```python
from build123d import *

# Parameters (mm, degrees)
SKETCH_1_W      = 60
SKETCH_1_H      = 60
EXTRUDE_1_DEPTH = 3
HOLE_WIZARD_1_D = 3
SKETCH_5_W      = 2
SKETCH_5_H      = 60
EXTRUDE_2_DEPTH = 23
SKETCH_6_W      = 60
SKETCH_6_H      = 3
EXTRUDE_3_DEPTH = 7
HOLE_WIZARD_2_D = 3.5
EXTRUDE_4_DEPTH = 3
EXTRUDE_5_DEPTH = 3


with BuildPart() as part:
    # 草图1 → 凸台-拉伸1 (new body)
    with BuildSketch(Plane(origin=(0, 0, 0), x_dir=(1, 0, 0), z_dir=(0, 1, 0))):
        Rectangle(SKETCH_1_W, SKETCH_1_H)
    extrude(amount=EXTRUDE_1_DEPTH)

    # 孔1 (through all)
    with Locations(Plane(origin=(0, 3, 0), x_dir=(1, 0, 0), z_dir=(0, 1, 0))):
        with Locations((-21.5, 21.5), (21.5, 21.5), (-21.5, -21.5), (21.5, -21.5)):
            Hole(HOLE_WIZARD_1_D / 2)

    # 草图5 → 凸台-拉伸2 (add)
    with BuildSketch(Plane(origin=(0, 3, 0), x_dir=(1, 0, 0), z_dir=(0, 1, 0))):
        with Locations((29, 0)):
            Rectangle(SKETCH_5_W, SKETCH_5_H)
        with Locations((-29, 0)):
            Rectangle(SKETCH_5_W, SKETCH_5_H)
    extrude(amount=EXTRUDE_2_DEPTH)

    # 草图6 → 凸台-拉伸3 (add)
    with BuildSketch(Plane(origin=(30, 0, 0), x_dir=(0, 0, -1), z_dir=(1, 0, 0))):
        with Locations((0, 24.5)):
            Rectangle(SKETCH_6_W, SKETCH_6_H)
    extrude_3 = extrude(amount=EXTRUDE_3_DEPTH)

    # 孔2 (through all)
    with Locations(Plane(origin=(0, 26, 0), x_dir=(1, 0, 0), z_dir=(0, 1, 0))):
        with Locations((33.5, 25), (33.5, -25)):
            hole_wizard_2 = Hole(HOLE_WIZARD_2_D / 2)

    # 镜向1: 凸台-拉伸3, 孔2 across plane
    add(extrude_3.mirror(Plane.ZY))
    add(hole_wizard_2.mirror(Plane.ZY), mode=Mode.SUBTRACT)

    # 草图11 → 凸台-拉伸4 (add)
    with BuildSketch(Plane(origin=(0, 0, -30), x_dir=(-1, 0, 0), z_dir=(0, 0, -1))):
        Polygon((-37, 26), (-28, 26), (-28, 3), (28, 3), (28, 26), (37, 26), (37, 23), (30, 23), (30, 0), (-30, 0), (-30, 23), (-37, 23), align=None)
    extrude(amount=EXTRUDE_4_DEPTH)

    # 草图12 → 凸台-拉伸5 (add)
    with BuildSketch(Plane(origin=(0, 0, -33), x_dir=(-1, 0, 0), z_dir=(0, 0, -1))):
        Polygon((-28, 18), (-13, 3), (-28, 3), align=None)
        Polygon((28, 18), (13, 3), (28, 3), align=None)
    extrude(amount=-EXTRUDE_5_DEPTH)


solid = part.part
```
CAD build for the part. Positions are in the model's coordinates, mm. A direction names the side the tool comes from. Round coordinates to 2 decimals unless told otherwise and drop trailing zeros. Write each loop counter-clockwise with the first axis right and the second up, starting at its lowest first coordinate (ties: lowest second). Pieces come first, ordered by that corner, then holes. Notation, with made-up numbers: (48.25, 75) - (107.25, 75) arc R22 ccw to (107.25, 114) - close; hole circle Ø7 at (-38.75, 89). An arc over 180 degrees is marked (long way). Write item = value, one per line. Start each with the question number.
Q1. Mould opens along X. For faces 6 (the flat face through (28, 15, -1)), 7 (the flat face through (-30, 12, -1)), 8 (the flat face through (33, 26, -1)), 9 (the flat face through (24, 7, -30)) say: pulls with the +X half, pulls with the -X half, needs draft (parallel to the pull), parting line crosses it, or undercut.
Q2. Band-saw the part on B-B (x = -21.5). Give the cut face in (y, z), then the cut area to 4 significant figures.
Q3. Which spindle directions (+Z, -Z, +X, -X, +Y, -Y) get a long thin tool onto all of the face, cutting with end or side? Do faces 1 (the flat face through (-24, 7, -30)), 2 (the cylindrical face through (-20.39, 1.48, -22.51)), 3 (the flat face through (-32, 26, -1)), 4 (the flat face through (33, 23, -1)), 5 (the flat face through (21, 11, -32)). Say none if no direction does.
Q4. Band-saw the part on A-A (y = 15.5). Give the cut face in (x, z).
Q5. Band-saw the part on C-C (z = -25). Give the cut face in (x, y).
Q6. Band-saw the part on D-D (z = -18). Give the cut face in (x, y).
Q7. Drop flat-ended pins along their axis: pin 1 (4.5 mm diameter, centred on x = -33.5, z = 25, fed in from +Y); pin 2 (4.5 mm diameter, centred on x = 23.5, y = 11.5, fed in from +Z); pin 3 (1.8 mm diameter, centred on x = -21.5, z = -21.5, fed in from +Y); pin 4 (5 mm diameter, centred on x = -21.5, z = 21.5, fed in from +Y). Give the stop position or say it passes through.
Q8. Probe L1, parallel to X at y = 1.15, z = -21.5; L2, parallel to Z at x = -33.5, y = 24.1; L3, parallel to Z at x = -21.5, y = 2.45. List the from-to ranges inside material, lowest first. Write a range as from..to.
Answers below:
q1.face_6 = undercut
q1.face_7 = pulls with the -X half
q1.face_8 = needs draft
q1.face_9 = undercut
q2.outline = (0, -33) - (11.5, -33) - (11.5, -30) - (3, -30) - (3, -23) - (0, -23) - close; (0, -20) - (3, -20) - (3, 20) - (0, 20) - close; (0, 23) - (3, 23) - (3, 30) - (0, 30) - close
q2.area = 196.5 mm2
q3.face_1 = +Z, +Y
q3.face_2 = +Y, -Y
q3.face_3 = +Z, -Z, +X, -X, +Y
q3.face_4 = +Z, -Z, +X, -Y
q3.face_5 = +Z, -Z, +Y
q4.outline = (-30, -33) - (-25.5, -33) - (-25.5, -30) - (-28, -30) - (-28, 30) - (-30, 30) - close; (25.5, -33) - (30, -33) - (30, 30) - (28, 30) - (28, -30) - (25.5, -30) - close
q5.outline = (-37, 23) - (-35.25, 23) - (-35.25, 26) - (-37, 26) - close; (-31.75, 23) - (-30, 23) - (-30, 0) - (30, 0) - (30, 23) - (31.75, 23) - (31.75, 26) - (28, 26) - (28, 3) - (-28, 3) - (-28, 26) - (-31.75, 26) - close; (35.25, 23) - (37, 23) - (37, 26) - (35.25, 26) - close
q6.outline = (-37, 23) - (-30, 23) - (-30, 0) - (30, 0) - (30, 23) - (37, 23) - (37, 26) - (28, 26) - (28, 3) - (-28, 3) - (-28, 26) - (-37, 26) - close
q7.pin_1 = 26
q7.pin_2 = -30
q7.pin_3 = through
q7.pin_4 = 3
q8.L1 = -30..-23, -20..20, 23..30
q8.L2 = -33..-26.75, -23.25..23.25, 26.75..30
q8.L3 = -33..-23, -20..20, 23..30
